Here's how the part is built. I have some questions about the finished solid (model axes, mm). Coordinates: 2 decimals unless noted, no trailing zeros. Write each loop counter-clockwise with the first axis right and the second up, starting at its lowest first coordinate (ties: lowest second). Pieces come first, ordered by that corner, then holes. Notation, with made-up numbers: M 69,23 L 110,23 A20 cw 110,30 Z; hole C 43.25,80 d7. An arc over 180 degrees is marked long. Use one line per item in the form item = value. Start each with the question number.
1. I want a section at D-D, the plane z = -1.5. List the corners of the cut face in (x, y) for me.
2. I'm going to push flat-ended pins straight in: pin 1 Ø1 at (y, z) = (-16, -0.5) entering from +X; pin 2 Ø14.5 at (x, y) = (20, -20) entering from +Z; pin 3 Ø1 at (x, z) = (92, -1.5) entering from +Y; pin 4 Ø8 at (x, y) = (100, -100) entering from +Z. Where does each tip first touch, or does it pass through?
3. I want a section at A-A, the plane y = -100. List the corners of the cut face in (x, z) for me.
4. Thinking about a two-plate mould opening in Y: for faces 1 (the face through (20.59, -104.46, -0.99)), 2 (the face through (48, -61, 0)), 3 (the face through (100.3, -40.6, -1)), 4 (the face through (103.32, -103.04, -0.99)), which applies, released by +Y, released by -Y, zero draft, split by the parting line, or undercut?
5. I want a section at C-C, the plane x = 20. List the corners of the cut face in (y, z) for me.
6. Please list where these lines run through material, in increasing order: line 1 along X through (y, z) = (-23, -1.8); line 2 along X through (y, z) = (-100, -1.25); line 3 along X through (y, z) = (-20, -0.55). Write a range as [from, to].
7. I want a section at B-B, the plane y = -60. List the corners of the cut face in (x, z) for me.
from build123d import *

# Parameters (mm, degrees)
EXTRUDE_1_DEPTH   = 2
HOLE_WIZARD_M81_D = 9
CHAMFER_1_SIZE    = 2


with BuildPart() as part:
    # Эскиз1 → Бобышка-Вытянуть1 (new body)
    with BuildSketch(Plane(origin=(0, 0, 0), x_dir=(1, 0, 0), z_dir=(0, 0, -1))):
        Polygon((0, 0), (0, 120), (120, 120), (120, 80), (80, 0), align=None)
    extrude(amount=EXTRUDE_1_DEPTH)

    # Отверстие с зазором M81 (through all)
    with Locations(Plane(origin=(0, 0, -2), x_dir=(1, 0, 0), z_dir=(0, 0, -1))):
        with Locations((60, 100), (20, 100), (20, 60), (20, 20), (100, 100), (60, 60), (60, 20)):
            Hole(HOLE_WIZARD_M81_D / 2)

    # Фаска1
    chamfer_1_edges = [part.edges().sort_by_distance(p)[0] for p in [
        (0, 0, -1),
        (0, -120, -1),
        (120, -120, -1),
    ]]
    chamfer(chamfer_1_edges, length=CHAMFER_1_SIZE)


solid = part.part
Answer list:
q1.outline = M 0,-118 L 2,-120 L 118,-120 L 120,-118 L 120,-80 L 80,0 L 2,0 L 0,-2 Z; hole C 20,-100 d9; hole C 20,-60 d9; hole C 20,-20 d9; hole C 60,-100 d9; hole C 60,-60 d9; hole C 60,-20 d9; hole C 100,-100 d9
q2.pin_1 = 88.25
q2.pin_2 = 0
q2.pin_3 = -23
q2.pin_4 = through
q3.outline = M 0,-2 L 15.5,-2 L 15.5,0 L 0,0 Z; M 24.5,-2 L 55.5,-2 L 55.5,0 L 24.5,0 Z; M 64.5,-2 L 95.5,-2 L 95.5,0 L 64.5,0 Z; M 104.5,-2 L 120,-2 L 120,0 L 104.5,0 Z
q4.face_1 = undercut
q4.face_2 = zero draft
q4.face_3 = released by +Y
q4.face_4 = undercut
q5.outline = M -120,-2 L -104.5,-2 L -104.5,0 L -120,0 Z; M -95.5,-2 L -64.5,-2 L -64.5,0 L -95.5,0 Z; M -55.5,-2 L -24.5,-2 L -24.5,0 L -55.5,0 Z; M -15.5,-2 L 0,-2 L 0,0 L -15.5,0 Z
q6.line_1 = [0, 16.65], [23.35, 56.65], [63.35, 91.5]
q6.line_2 = [0, 15.5], [24.5, 55.5], [64.5, 95.5], [104.5, 120]
q6.line_3 = [0, 15.5], [24.5, 55.5], [64.5, 90]
q7.outline = M 0,-2 L 15.5,-2 L 15.5,0 L 0,0 Z; M 24.5,-2 L 55.5,-2 L 55.5,0 L 24.5,0 Z; M 64.5,-2 L 110,-2 L 110,0 L 64.5,0 Z
